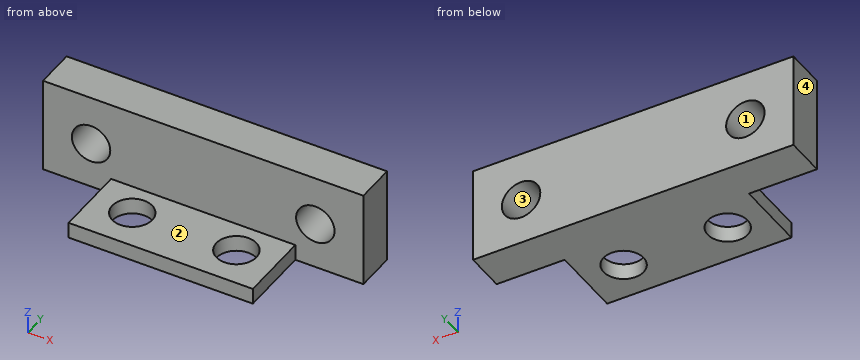
from build123d import *

# Parameters (mm, degrees)
BOSS_EXTRU_1_DEPTH      = 40
ESQUISSE2_R             = 2.4
ENL_V_MAT_EXTRU_1_DEPTH = 40
ESQUISSE3_W             = 8.5
ESQUISSE3_H             = 9
ENL_V_MAT_EXTRU_2_DEPTH = 40
ESQUISSE4_R             = 2.5
ENL_V_MAT_EXTRU_3_DEPTH = 40


with BuildPart() as part:
    # Esquisse1 → Boss.-Extru.1 (new body)
    with BuildSketch(Plane(origin=(0, 0, 0), x_dir=(0, 0, -1), z_dir=(1, 0, 0))):
        Polygon((0, 0), (0, 14), (-12, 14), (-12, 9), (-2, 9), (-2, 0), align=None)
    extrude(amount=BOSS_EXTRU_1_DEPTH)

    # Esquisse2 → Enlèv. mat.-Extru.1 (cut)
    with BuildSketch(Plane(origin=(0, 14, 0), x_dir=(1, 0, 0), z_dir=(0, 1, 0))):
        with Locations(Location((34, -5.8, 0), (0, 0, 270))):  # turned: the seam where the file's is
            Circle(ESQUISSE2_R)
        with Locations(Location((6, -5.8, 0), (0, 0, 270))):  # turned: the seam where the file's is
            Circle(ESQUISSE2_R)
    extrude(amount=-ENL_V_MAT_EXTRU_1_DEPTH, mode=Mode.SUBTRACT)

    # Esquisse3 → Enlèv. mat.-Extru.2 (cut)
    with BuildSketch(Plane.XY.offset(2)):
        with Locations((4.25, 4.5)):
            Rectangle(ESQUISSE3_W, ESQUISSE3_H)
        with Locations((35.75, 4.5)):
            Rectangle(ESQUISSE3_W, ESQUISSE3_H)
    extrude(amount=-ENL_V_MAT_EXTRU_2_DEPTH, mode=Mode.SUBTRACT)

    # Esquisse4 → Enlèv. mat.-Extru.3 (cut)
    with BuildSketch(Plane.XY.offset(2)):
        with Locations((26.5, 5)):
            Circle(ESQUISSE4_R)
        with Locations((13.5, 5)):
            Circle(ESQUISSE4_R)
    extrude(amount=-ENL_V_MAT_EXTRU_3_DEPTH, mode=Mode.SUBTRACT)


solid = part.part
Work out the finished part from the listing and answer in its coordinate system (mm). Face numbers are marked on the shaded views. Give positions to 0.01 mm unless a question says otherwise; leave off trailing zeros. Order: outer loops, then holes, each group sorted by start corner. A loop starts at its lowest first (then second) coordinate and runs counter-clockwise, first axis right, second up. Notation, with made-up numbers: (33.25, 42.25) -> (66.25, 42.25) arc R22 ccw to (66.25, 72.25) -> close; hole circle Ø3 at (83, 16). An arc over 180 degrees is marked (long way). Answer as a JSON object with one key per item and string values. Group by question number.
1. The mould has two halves that part along X. Classify the marked faces 1, 2, 3 and 4: released by +X, released by -X, zero draft, split by the parting line, or undercut.
2. Section C-C on y = 5 is taken. Determine the outline of the cut face in (x, z), plus the area to 3 significant figures.
3. Section B-B on z = 5.8 is taken. Determine the outline of the cut face in (x, y), plus the area to 3 significant figures.
4. Section D-D on y = 9.5 is taken. Determine the outline of the cut face in (x, z), plus the area to 3 significant figures.
5. Consider line 1 along X through (y, z) = (10.4, 5.8); line 2 along Y through (x, z) = (26.5, 0.55); line 3 along Z through (x, y) = (22.5, 8). Determine where each line is inside the solid, lowest interval first. Write a range as [from, to].
6. Section A-A on x = 34 is taken. Determine the outline of the cut face in (y, z), plus the area to 3 significant figures.
7. Flat-ended cylindrical pins translate along their axes: pin 1 Ø1 at (x, z) = (19, 9) entering from -Y; pin 2 Ø0.6 at (y, z) = (3, 1) entering from +X; pin 3 Ø2.5 at (x, y) = (19.5, 6.5) entering from +Z. Find the tip coordinate at first contact, or state that the pin passes through.
Result sheet:
{
 "1": {"face 1": "undercut", "face 2": "zero draft", "face 3": "undercut", "face 4": "released by -X"},
 "2": {"outline": "(8.5, 0) -> (11, 0) -> (11, 2) -> (8.5, 2) -> close; (16, 0) -> (24, 0) -> (24, 2) -> (16, 2) -> close; (29, 0) -> (31.5, 0) -> (31.5, 2) -> (29, 2) -> close", "area": "26.0 mm^2"},
 "3": {"outline": "(0, 9) -> (3.6, 9) -> (3.6, 14) -> (0, 14) -> close; (8.4, 9) -> (31.6, 9) -> (31.6, 14) -> (8.4, 14) -> close; (36.4, 9) -> (40, 9) -> (40, 14) -> (36.4, 14) -> close", "area": "152 mm^2"},
 "4": {"outline": "(0, 0) -> (40, 0) -> (40, 12) -> (0, 12) -> close; hole circle Ø4.8 at (6, 5.8); hole circle Ø4.8 at (34, 5.8)", "area": "444 mm^2"},
 "5": {"line 1": "x = [0, 3.6], [8.4, 31.6], [36.4, 40]", "line 2": "y = [0, 2.5], [7.5, 14]", "line 3": "z = [0, 2]"},
 "6": {"outline": "(9, 0) -> (14, 0) -> (14, 3.4) -> (9, 3.4) -> close; (9, 8.2) -> (14, 8.2) -> (14, 12) -> (9, 12) -> close", "area": "36.0 mm^2"},
 "7": {"pin 1": "stops at y = 9", "pin 2": "stops at x = 31.5", "pin 3": "stops at z = 2"}
}
